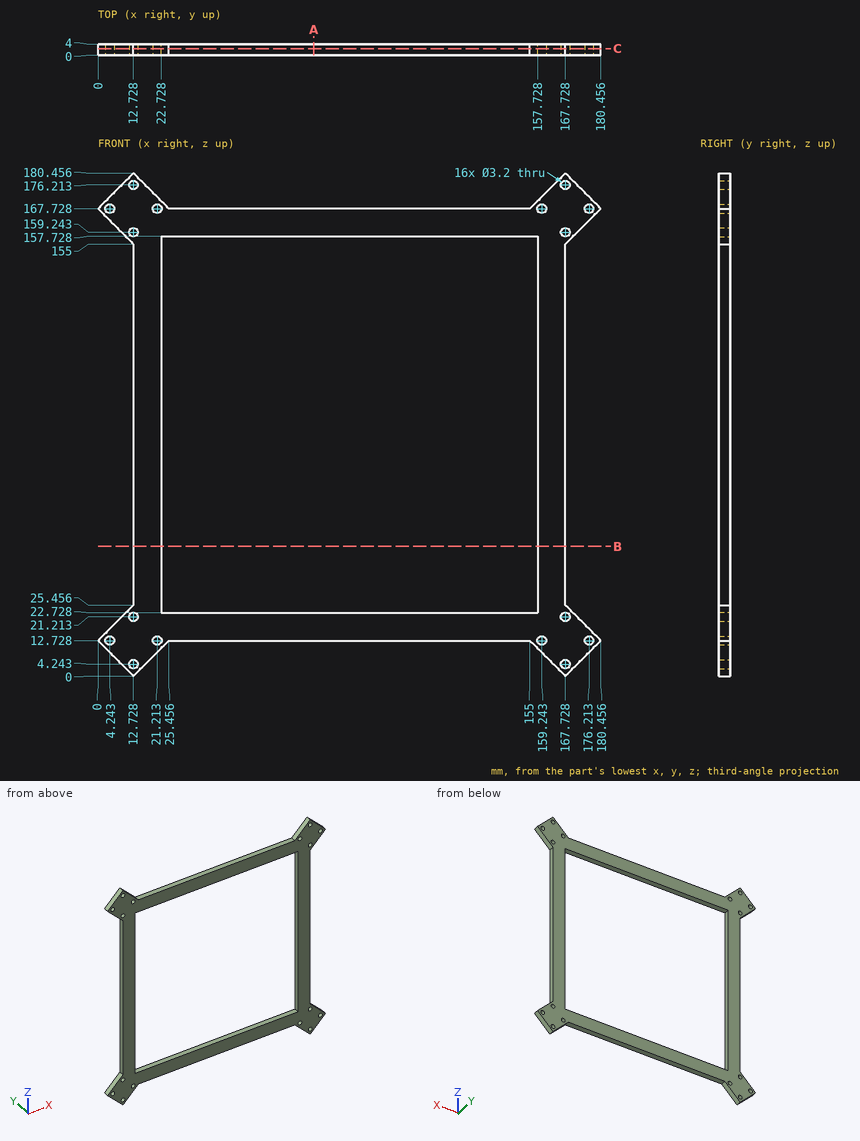
Here's the drawing with two shaded views (mm, measured from the low corner). I have some questions. Give positions to 0.01 mm unless a question says otherwise; leave off trailing zeros. Order: outer loops, then holes, each group sorted by start corner. A loop starts at its lowest first (then second) coordinate and runs counter-clockwise, first axis right, second up. Notation, with made-up numbers: M -6,13.5 L 43,13.5 A28 cw 43,38.5 Z; hole C 82.5,67 d5. An arc over 180 degrees is marked long. Answer as a JSON object with one key per item and string values. Group by question number.
1) I'm going to push flat-ended pins straight in: pin 1 Ø2 at (y, z) = (1.5, 91) entering from +X; pin 2 Ø1.2 at (y, z) = (1.5, 93.5) entering from -X; pin 3 Ø2 at (x, y) = (41, 1.5) entering from +Z; pin 4 Ø4 at (x, z) = (21.21, 12.73) entering from +Y. Where does each tip first touch, or does it pass through?
2) Please list where these lines run through material, in increasing order: L1, parallel to Z at x = 84, y = 1.65; L2, parallel to X at y = 1.85, z = 160. Write a range as [from, to].
3) Suppose I cut it at C-C, the plane y = 2.3. Count the separate pieces of the cut face and the enclosed holes in it, plus the area to 3 significant figures.
4) Suppose I cut it at A-A, the plane x = 77.5. Write out the boundary of the cut face in (y, z), plus the area to 3 significant figures.
5) Suppose I cut it at B-B, the plane z = 46.5. Write out the boundary of the cut face in (x, y).
Results found:
{
 "1": {"pin 1": "x = 167.73", "pin 2": "x = 12.73", "pin 3": "z = 167.73", "pin 4": "y = 4"},
 "2": {"L1": "[12.73, 22.73], [157.73, 167.73]", "L2": "[7.73, 11.32], [14.14, 166.32], [169.14, 172.73]"},
 "3": {"separate pieces": "1", "enclosed holes": "17", "area": "6,640 mm²"},
 "4": {"outline": "M 0,12.73 L 4,12.73 L 4,22.73 L 0,22.73 Z; M 0,157.73 L 4,157.73 L 4,167.73 L 0,167.73 Z", "area": "80.0 mm²"},
 "5": {"outline": "M 12.73,0 L 22.73,0 L 22.73,4 L 12.73,4 Z; M 157.73,0 L 167.73,0 L 167.73,4 L 157.73,4 Z"}
}
